```python
from build123d import *

# Parameters (mm, degrees)
ESTRUSIONE1_DEPTH                                    = 30
ESTRUSIONE2_DEPTH                                    = 14
RIPETIZIONE_A_L1_COUNT                               = 2
RIPETIZIONE_A_L1_PITCH                               = 220
RIPETIZIONE_A_L1_COUNT_DIR2                          = 2
RIPETIZIONE_A_L1_PITCH_DIR2                          = 126
SCHIZZO3_R                                           = 45
ESTRUSIONE3_DEPTH                                    = 5
M10_LAMATURA_PER_VITE_A_COPERTURA_CILIND_D           = 11
M10_LAMATURA_PER_VITE_A_COPERTURA_CILIND_CBORE_D     = 18
M10_LAMATURA_PER_VITE_A_COPERTURA_CILIND_CBORE_DEPTH = 10
M10_TAPPED_HOLE1_D                                   = 8.5
M10_TAPPED_HOLE1_DEPTH                               = 25
M10_TAPPED_HOLE1_TIP                                 = 2.553657631


with BuildPart() as part:
    # Schizzo1 → Estrusione1 (new body)
    with BuildSketch(Plane(origin=(0, 0, 0), x_dir=(1, 0, 0), z_dir=(0, 1, 0))):
        Polygon((-14, 91.5), (-14, 48.5), (0, 43.5), (0, 0), (280, 0), (280, 40.5), (264, 45.5), (264, 94.5), (280, 99.5), (280, 140), (0, 140), (0, 96.5), align=None)
    extrude(amount=ESTRUSIONE1_DEPTH)

    # Schizzo2 → Estrusione2 (cut)
    with BuildSketch(Plane.XY):
        with BuildLine():
            Line((22, 12), (22, 0))
            Line((22, 0), (38, 0))
            Line((38, 0), (38, 12))
            ThreePointArc((38, 12), (30, 20), (22, 12))
        make_face()
    estrusione2 = extrude(amount=-ESTRUSIONE2_DEPTH, mode=Mode.SUBTRACT)

    # Ripetizione a L1: Estrusione2 2 × 2
    with Locations(*[(i * RIPETIZIONE_A_L1_PITCH, 0, -j * RIPETIZIONE_A_L1_PITCH_DIR2) for i in range(RIPETIZIONE_A_L1_COUNT) for j in range(RIPETIZIONE_A_L1_COUNT_DIR2) if (i, j) != (0, 0)]):
        add(estrusione2, mode=Mode.SUBTRACT)

    # Schizzo3 → Estrusione3 (cut)
    with BuildSketch(Plane(origin=(0, 30, 0), x_dir=(1, 0, 0), z_dir=(0, 1, 0))):
        with Locations(Location((68, 70, 0), (0, 0, 270))):
            Circle(SCHIZZO3_R)
        with Locations(Location((209, 70, 0), (0, 0, 270))):
            Circle(SCHIZZO3_R)
    extrude(amount=-ESTRUSIONE3_DEPTH, mode=Mode.SUBTRACT)

    # M10 Lamatura per vite a copertura cilindrica esagonale2 (through all)
    with Locations(Plane.XZ):
        with Locations((68, -70), (209, -70)):
            CounterBoreHole(M10_LAMATURA_PER_VITE_A_COPERTURA_CILIND_D / 2, M10_LAMATURA_PER_VITE_A_COPERTURA_CILIND_CBORE_D / 2, M10_LAMATURA_PER_VITE_A_COPERTURA_CILIND_CBORE_DEPTH)

    # M10 Tapped Hole1
    with Locations(Plane.XZ):
        with Locations((93.5, -25), (183.5, -25), (93.5, -115), (183.5, -115)):
            Hole(M10_TAPPED_HOLE1_D / 2, depth=M10_TAPPED_HOLE1_DEPTH)
            with Locations((0, 0, -(M10_TAPPED_HOLE1_DEPTH + M10_TAPPED_HOLE1_TIP / 2))):  # 118° drill point
                Cone(0, M10_TAPPED_HOLE1_D / 2, M10_TAPPED_HOLE1_TIP, mode=Mode.SUBTRACT)


solid = part.part
```
Check sheet for the modelled part. Datum: model origin and axes. Units: mm. A direction names the side the tool comes from. Give positions to 0.01 mm unless a question says otherwise; leave off trailing zeros. Loops run counter-clockwise (first coordinate to the right, second up) from the corner with the lowest first, then second, coordinate; pieces in that order, holes last. Notation, with made-up numbers: M 51.5,56.25 L 70.5,56.25 A7 ccw 70.5,69.25 Z; hole C 59.5,86.5 d7. An arc over 180 degrees is marked long. Answer in a Markdown table with one row per item.
1) Thickness scan on line 1 (X direction, y = 8.25, z = -115); line 2 (X direction, y = 28, z = -69.5); line 3 (Z direction, x = 209, y = 15.5). Record the ranges inside material, lowest first.
Solutions:
| item | result |
|---|---|
| line 1 | x = 0 to 89.25, 97.75 to 179.25, 187.75 to 280 |
| line 2 | x = -14 to 23, 113 to 164, 254 to 264 |
| line 3 | z = -140 to -75.5, -64.5 to 0 |
2) Tool access check on faces 4 (the face through (186.87, 12.67, -27.59)), 5 (the face through (242, 6, -133)), 6 (the face through (24.07, 27.54, -79.76)), 7 (the face through (258, 6, -7)), 8 (the face through (0, 15, -22)). Record the directions out of +Z, -Z, +X, -X, +Y, -Y that give a thin tool (end or side, any length) a straight path to the whole face; none if there is none.
Solutions:
| item | result |
|---|---|
| face 4 | -Y |
| face 5 | -Z, -Y |
| face 6 | +Y |
| face 7 | +Z, -Y |
| face 8 | +Z, -X, +Y, -Y |
3) Depth check by flat-ended pin: pin 1 (16 mm diameter, centred on x = 209, z = -70, fed in from +Y); pin 2 (5 mm diameter, centred on x = 26, y = 12.5, fed in from +Z). Enter the tip coordinate at first touch or a pass-through.
Solutions:
| item | result |
|---|---|
| pin 1 | stops at y = 25 |
| pin 2 | stops at z = -14 |
4) Cross-section at A-A (z = -70). Enter the section's corners in (x, y).
Solutions:
| item | result |
|---|---|
| outline | M -14,0 L 59,0 L 59,10 L 62.5,10 L 62.5,25 L 23,25 L 23,30 L -14,30 Z; M 73.5,10 L 77,10 L 77,0 L 200,0 L 200,10 L 203.5,10 L 203.5,25 L 164,25 L 164,30 L 113,30 L 113,25 L 73.5,25 Z; M 214.5,10 L 218,10 L 218,0 L 264,0 L 264,30 L 254,30 L 254,25 L 214.5,25 Z |
5) Cross-section at D-D (x = 52.5). Enter the section's corners in (y, z), plus the area to 3 significant figures.
Solutions:
| item | result |
|---|---|
| outline | M 0,-140 L 30,-140 L 30,-112.25 L 25,-112.25 L 25,-27.75 L 30,-27.75 L 30,0 L 0,0 Z |
| area | 3,780 mm^2 |
6) Mould release check, pull along Z, two halves, no side actions. Record for faces 1 (the face through (200, 25, -71)), 2 (the face through (30, 20, -133)), 3 (the face through (142, 15, -140)): released by +Z, released by -Z, zero draft, split by the parting line, or undercut.
Solutions:
| item | result |
|---|---|
| face 1 | undercut |
| face 2 | zero draft |
| face 3 | released by -Z |
7) Cross-section at C-C (y = 3.5). Count the separate pieces of the cut face and the enclosed holes in it, plus the area to 3 significant figures.
Solutions:
| item | result |
|---|---|
| separate pieces | 1 |
| enclosed holes | 6 |
| area | 37,400 mm^2 |
8) Cross-section at B-B (x = 209). Enter the section's corners in (y, z), plus the area to 4 significant figures.
Solutions:
| item | result |
|---|---|
| outline | M 0,-140 L 30,-140 L 30,-115 L 25,-115 L 25,-75.5 L 10,-75.5 L 10,-79 L 0,-79 Z; M 0,-61 L 10,-61 L 10,-64.5 L 25,-64.5 L 25,-25 L 30,-25 L 30,0 L 0,0 Z |
| area | 3,405 mm^2 |
